For this review, take the finished solid that the model builds, in its own axes (mm). A direction names the side the tool comes from. Round coordinates to 2 decimals unless told otherwise and drop trailing zeros. Write each loop counter-clockwise with the first axis right and the second up, starting at its lowest first coordinate (ties: lowest second). Pieces come first, ordered by that corner, then holes. Notation, with made-up numbers: M 82,15 L 121,15 A14 ccw 121,34 Z; hole C -22,46 d9. An arc over 180 degrees is marked long. Answer in a Markdown table with one row per item.
```python
from build123d import *

# Parameters (mm, degrees)
F1_DEPTH = 3.175


with BuildPart() as f1:
    # F0 (on Top) → F1 (new body)
    with BuildSketch(Plane.XY):
        with BuildLine():
            Line((25.241197, 4.974793), (3.295561, 4.974793))
            Line((3.295561, 4.974793), (3.295561, 8.149793))
            Line((3.295561, 8.149793), (-1.704439, 8.149793))
            Line((-1.704439, 8.149793), (-6.704439, 8.149793))
            Line((-6.704439, 8.149793), (-6.704439, 4.974793))
            Line((-6.704439, 4.974793), (-28.650075, 4.974793))
            Line((-28.650075, 4.974793), (-23.579421, -9.504047))
            ThreePointArc((-23.579421, -9.504047), (-21.753258, -11.929592), (-18.86044, -12.851406))
            Line((-18.86044, -12.851406), (-1.704439, -12.851406))
            Line((-1.704439, -12.851406), (15.451562, -12.851406))
            ThreePointArc((15.451562, -12.851406), (18.34438, -11.929592), (20.170542, -9.504047))
            Line((20.170542, -9.504047), (25.241197, 4.974793))
        make_face()
        with BuildLine():
            ThreePointArc((18.575678, -0.025208), (19.840188, -0.678574), (20.038877, -2.08797))
            Line((20.038877, -2.08797), (18.505102, -6.467537))
            ThreePointArc((18.505102, -6.467537), (16.67894, -8.893082), (13.786122, -9.814896))
            Line((13.786122, -9.814896), (-17.195, -9.814896))
            ThreePointArc((-17.195, -9.814896), (-20.087818, -8.893082), (-21.913981, -6.467537))
            Line((-21.913981, -6.467537), (-23.447755, -2.08797))
            ThreePointArc((-23.447755, -2.08797), (-23.249066, -0.678574), (-21.984557, -0.025208))
            Line((-21.984557, -0.025208), (18.575678, -0.025208))
        make_face(mode=Mode.SUBTRACT)
    extrude(amount=F1_DEPTH)


solid = f1.part
```
Q1. Mouldability with a two-part tool opening along Y and no side actions: class faces 4 (the face through (-2, 8.15, 2)), 5 (the face through (-2.08, 0.13, 3.175)), 6 (the face through (19.3, -4.2, 1.6)), 7 (the face through (-22.67, -4.31, 1.57)) as +Y half, -Y half, draft (parallel to the pull), parting line (faces both ways), or undercut.
Found:
| item | result |
|---|---|
| face 4 | +Y half |
| face 5 | draft |
| face 6 | undercut |
| face 7 | undercut |
Q2. Take a section at B-B (x = -5). State the section outline as (y, z) points (3 decimals).
Found:
| item | result |
|---|---|
| outline | M -12.851,0 L -9.815,0 L -9.815,3.175 L -12.851,3.175 Z; M -0.025,0 L 8.15,0 L 8.15,3.175 L -0.025,3.175 Z |
Q3. Take a section at C-C (y = -8). State the section outline as (x, z) points (3 decimals), then the cut area to 3 significant figures.
Found:
| item | result |
|---|---|
| outline | M -24.106,0 L -21.049,0 L -21.049,3.175 L -24.106,3.175 Z; M 17.64,0 L 20.697,0 L 20.697,3.175 L 17.64,3.175 Z |
| area | 19.4 mm² |
Q4. Take a section at A-A (z = 2.7). State the section outline as (x, y) points (3 decimals).
Found:
| item | result |
|---|---|
| outline | M -28.65,4.975 L -23.579,-9.504 A5 ccw -18.86,-12.851 L 15.452,-12.851 A5 ccw 20.171,-9.504 L 25.241,4.975 L 3.296,4.975 L 3.296,8.15 L -6.704,8.15 L -6.704,4.975 Z; hole M -23.448,-2.088 L -21.914,-6.468 A5 ccw -17.195,-9.815 L 13.786,-9.815 A5 ccw 18.505,-6.468 L 20.039,-2.088 A1.55 ccw 18.576,-0.025 L -21.985,-0.025 A1.55 ccw Z |
Q5. Take a section at D-D (y = 2.5). State the section outline as (x, z) points (1 decimal), then the cut area to 3 significant figures.
Found:
| item | result |
|---|---|
| outline | M -27.8,0 L 24.4,0 L 24.4,3.2 L -27.8,3.2 Z |
| area | 166 mm² |
Q6. For probe 1 along Y at (x, z) = (-2.5, 2.25); probe 2 along Y at (x, z) = (10.5, 1.45); probe 3 along X at (y, z) = (5.75, 2.5), list the stretches that pass through material, from the lowest coordinate up.
Found:
| item | result |
|---|---|
| probe 1 | -12.85 to -9.81, -0.03 to 8.15 |
| probe 2 | -12.85 to -9.81, -0.03 to 4.97 |
| probe 3 | -6.7 to 3.3 |
Q7. Machinability: for faces 1 (the face through (3.296, 7, 2)), 2 (the face through (-23.261, -0.696, 1.565)), 3 (the face through (-6.704, 7, 2)), which of the approach directions +Z, -Z, +X, -X, +Y, -Y give a long, thin tool a straight path to every point of the face, cutting with its end or side? Answer none if there is none.
Found:
| item | result |
|---|---|
| face 1 | +Z, -Z, +X, +Y |
| face 2 | +Z, -Z |
| face 3 | +Z, -Z, -X, +Y |
Q8. Insertion check: P1, Ø1, axis at y = -8.5, z = 1, coming from the +X side; P2, Ø1, axis at y = -2.5, z = 1, coming from the -X side; P3, Ø1, axis at y = 6.5, z = 1.5, coming from the +X side. Each pin has a flat end and moves straight along its axis. Give the tip position at first contact, or say it passes through.
Found:
| item | result |
|---|---|
| P1 | x = 20.7 |
| P2 | x = -26.21 |
| P3 | x = 3.3 |
